Autodesk Inventor part; units mm, degrees
ref_plane "YZ Plane" through (0, 0, 0) normal (1, 0, 0) x (0, 1, 0)
ref_plane "XZ Plane" through (0, 0, 0) normal (0, 1, 0) x (-1, 0, 0)
ref_plane "XY Plane" through (0, 0, 0) normal (0, 0, 1) x (1, 0, 0)
sketch "Эскиз1" plane through (0, 0, 0) normal (0, 1, 0) x (-1, 0, 0)
  circle A0 centre (0, 0) radius 2.75
  circle A1 centre (0, 0) radius 5.5
  dimension "d0" = 5.5
  dimension "d1" = 11
extrude "Выдавливание1" add sketch "Эскиз1" along normal blind 7.6
fillet "Сопряжение1" radius 0.8 2 edges at (5.5, 7.6, 0) (5.5, 0, 0)
chamfer "Фаска1" distance 0.6 angle 45 2 edges at (2.75, 7.6, 0) (2.75, 0, 0)
properties part number "prostavka_7,6"
Geometry: final body of the model. Coordinates: model frame, mm. Give positions to 0.01 mm unless a question says otherwise; leave off trailing zeros. Loops run counter-clockwise (first coordinate to the right, second up) from the corner with the lowest first, then second, coordinate; pieces in that order, holes last. Notation, with made-up numbers: (2.25, -26.5) - (35.25, -26.5) arc R20 cw to (35.25, -20.5) - close; hole circle Ø8 at (44.25, 13). An arc over 180 degrees is marked (long way). Answer as CSV lines item,"result". Start each with the question number.
1. Section C-C, the plane y = 3.5. Return loops of the section in (x, z).
2. Section A-A, the plane z = 0. Return loops of the section in (x, y), plus the area to 3 significant figures.
3. Pin query (flat end, axial travel): P1, Ø1, axis at x = 2.5, z = 0.5, coming from the -Y side; P2, Ø1, axis at x = 1, y = 6.5, coming from the -Z side. Return the tip coordinate at first contact, or that it passes through.
4. Ray query, L1, parallel to Z at x = 0, y = 4; L2, parallel to X at y = 3, z = 2.25; L3, parallel to X at y = 4, z = -2. Return the intervals inside material, ascending.
5. Section B-B, the plane x = 0. Return loops of the section in (y, z), plus the area to 3 significant figures.
6. Draft query along Z for faces 1 (the face through (1.19, 3.76, 5.37)), 2 (the face through (-3, 0, -2)), 3 (the face through (0.596, 3.755, 2.685)). Return one class per face: released by +Z, released by -Z, zero draft, split by the parting line, or undercut.
Answers:
1,outline,"circle Ø11 at (0, 0); hole circle Ø5.5 at (0, 0)"
2,outline,"(-5.5, 0.8) arc R0.8 ccw to (-4.7, 0) - (-3.35, 0) - (-2.75, 0.6) - (-2.75, 7) - (-3.35, 7.6) - (-4.7, 7.6) arc R0.8 ccw to (-5.5, 6.8) - close; (2.75, 0.6) - (3.35, 0) - (4.7, 0) arc R0.8 ccw to (5.5, 0.8) - (5.5, 6.8) arc R0.8 ccw to (4.7, 7.6) - (3.35, 7.6) - (2.75, 7) - close"
2,area,"40.5 mm2"
3,P1,"stops at y = 0.3"
3,P2,"stops at z = -5.48"
4,L1,"z = -5.5 to -2.75, 2.75 to 5.5"
4,L2,"x = -5.02 to -1.58, 1.58 to 5.02"
4,L3,"x = -5.12 to -1.89, 1.89 to 5.12"
5,outline,"(0, -4.7) arc R0.8 ccw to (0.8, -5.5) - (6.8, -5.5) arc R0.8 ccw to (7.6, -4.7) - (7.6, -3.35) - (7, -2.75) - (0.6, -2.75) - (0, -3.35) - close; (0, 3.35) - (0.6, 2.75) - (7, 2.75) - (7.6, 3.35) - (7.6, 4.7) arc R0.8 ccw to (6.8, 5.5) - (0.8, 5.5) arc R0.8 ccw to (0, 4.7) - close"
5,area,"40.5 mm2"
6,face 1,"split by the parting line"
6,face 2,"zero draft"
6,face 3,"undercut"
